The figure shows three views and two pictorial views of one solid part (mm, origin at its lowest corner). Answer the questions. A direction names the side the tool comes from. Coordinates: 2 decimals unless noted, no trailing zeros. Write each loop counter-clockwise with the first axis right and the second up, starting at its lowest first coordinate (ties: lowest second). Pieces come first, ordered by that corner, then holes. Notation, with made-up numbers: M 52,86 L 106,86 A11 ccw 106,106 Z; hole C -15.5,-6 d2. An arc over 180 degrees is marked long. Use a Markdown table: item, result. Add a question column.
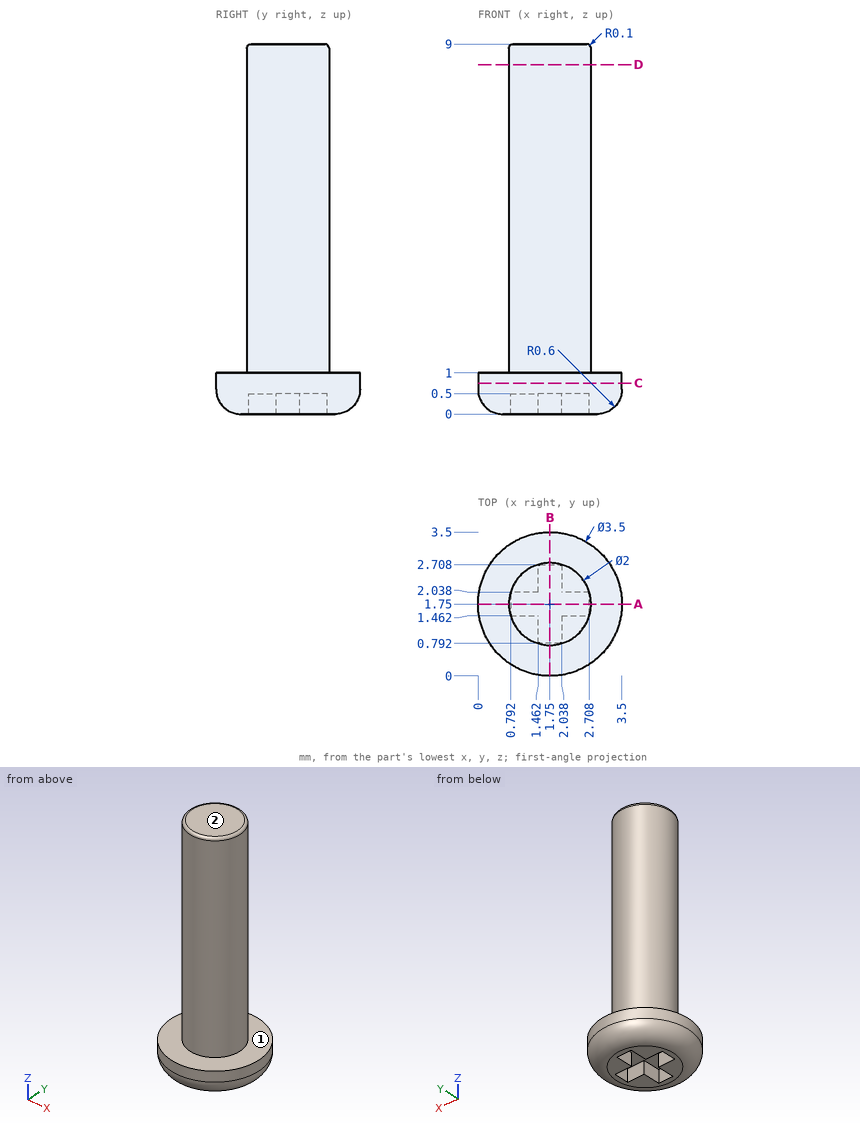
Item 1: Find section C-C on z = 0.75. Give the vertices of the cut face in (x, y).
Item 2: Find section D-D on z = 8.5. Give the vertices of the cut face in (x, y).
Item 3: Find section A-A on y = 1.75. Give the vertices of the cut face in (x, z).
Item 4: For the marked faces 1 and 2, determine the directions among +Z, -Z, +X, -X, +Y, -Y from which every point of the face is accessible in a straight line to the end or side of a thin tool.
Item 5: Consider probe 1 along Z at (x, y) = (2.2, 1.7); probe 2 along Z at (x, y) = (1.05, 0.95); probe 3 along X at (y, z) = (1.7, 5.5). Determine where each line is inside the solid, lowest interval first.
Item 6: Each of these flat-tipped pins is pushed along its axis until it touches: pin 1 (0.6 mm diameter, centred on y = 2.5, z = 0.5, fed in from +X); pin 2 (0.6 mm diameter, centred on x = 1.5, z = 0, fed in from -Y) (1 decimal); pin 3 (0.6 mm diameter, centred on x = 2.5, z = 0.5, fed in from +Y). Where does it stop, or does it pass through?
Geometry says:
| question | item | result |
|---|---|---|
| 1 | outline | C 1.75,1.75 d3.5 |
| 2 | outline | C 1.75,1.75 d2 |
| 3 | outline | M 0,0.6 A0.6 ccw 0.6,0 L 0.79,0 L 0.79,0.5 L 2.71,0.5 L 2.71,0 L 2.9,0 A0.6 ccw 3.5,0.6 L 3.5,1 L 2.75,1 L 2.75,8.9 A0.1 ccw 2.65,9 L 0.85,9 A0.1 ccw 0.75,8.9 L 0.75,1 L 0,1 Z |
| 4 | face 1 | +Z |
| 4 | face 2 | +Z, +X, -X, +Y, -Y |
| 5 | probe 1 | z = 0.5 to 9 |
| 5 | probe 2 | z = 0 to 1 |
| 5 | probe 3 | x = 0.75 to 2.75 |
| 6 | pin 1 | stops at x = 3.44 |
| 6 | pin 2 | stops at y = 0.1 |
| 6 | pin 3 | stops at y = 3.44 |
